from build123d import *

# Parameters (mm, degrees)
SKETCH1_R             = 11
EXTRUDE1_DEPTH        = 2.5
F_6_32_TAPPED_HOLE3_D = 2.7051
CHAMFER1_SIZE         = 0.254
SKETCH2_R             = 4
EXTRUDE2_DEPTH        = 6


with BuildPart() as part:
    # Sketch1 → Extrude1 (new body, symmetric)
    with BuildSketch(Plane.XY):
        Circle(SKETCH1_R)
    extrude(amount=EXTRUDE1_DEPTH, both=True)

    # #6-32 Tapped Hole3 (through all)
    with Locations(Plane(origin=(0, 7.599342077, 2.5), x_dir=(1, 0, 0), z_dir=(0, 0, 1))):
        with Locations((0, 0), (-7.599342077, -7.599342077), (7.599342077, -7.599342077), (0, -15.198684154)):
            Hole(F_6_32_TAPPED_HOLE3_D / 2)

    # Chamfer1
    chamfer1_edges = [part.edges().sort_by_distance(p)[0] for p in [
        (8.951892077, 0, 2.5),
        (8.951892077, 0, -2.5),
        (-6.246792077, 0, 2.5),
        (-6.246792077, 0, -2.5),
        (1.35255, 7.599342077, 2.5),
        (1.35255, 7.599342077, -2.5),
        (1.35255, -7.599342077, 2.5),
        (1.35255, -7.599342077, -2.5),
    ]]
    chamfer(chamfer1_edges, length=CHAMFER1_SIZE)

    # Sketch2 → Extrude2 (cut, through all)
    with BuildSketch(Plane.XY.offset(2.5)):
        Circle(SKETCH2_R)
    extrude(amount=-EXTRUDE2_DEPTH, mode=Mode.SUBTRACT)


solid = part.part
Read the model definition and answer for the solid it produces. Units are mm, in the model's axes. Round coordinates to 2 decimals unless told otherwise and drop trailing zeros. Write each loop counter-clockwise with the first axis right and the second up, starting at its lowest first coordinate (ties: lowest second). Pieces come first, ordered by that corner, then holes.
Q1. Find section C-C on y = -2.5. Determine the outline of the cut face in (x, z).
Values:
outline: (-10.71, -2.5) - (-3.12, -2.5) - (-3.12, 2.5) - (-10.71, 2.5) - close; (3.12, -2.5) - (10.71, -2.5) - (10.71, 2.5) - (3.12, 2.5) - close
Q2. The mould has two halves that part along Y. Classify faces 1 (the face through (-2.38, -10.74, 0.04)), 2 (the face through (0.29, 6.28, -0.03)), 3 (the face through (0, -5, 2.5)): released by +Y, released by -Y, zero draft, split by the parting line, or undercut.
Values:
face 1: split by the parting line
face 2: undercut
face 3: zero draft
Q3. Straight lines are drawn through the part: line 1 (Y direction, x = 0, z = 1.45); line 2 (Y direction, x = -7.5, z = -0.2); line 3 (Y direction, x = -1, z = 0.7). For each, find the intervals that lie inside material, in ascending order.
Values:
line 1: y = -11 to -8.95, -6.25 to -4, 4 to 6.25, 8.95 to 11
line 2: y = -8.05 to -1.35, 1.35 to 8.05
line 3: y = -10.95 to -8.51, -6.69 to -3.87, 3.87 to 6.69, 8.51 to 10.95
Q4. Flat-ended cylindrical pins translate along their axes: P1, Ø1, axis at y = -7.5, z = 0.5, coming from the +X side; P2, Ø1, axis at x = -8.5, y = 0, coming from the -Z side; P3, Ø3, axis at x = -7.6, y = 0, coming from the -Z side. Find the tip coordinate at first contact, or state that the pin passes through.
Values:
P1: stops at x = 8.49
P2: stops at z = -2.29
P3: stops at z = -2.39
Q5. Find section A-A on y = 0. Determine the outline of the cut face in (x, z).
Values:
outline: (-11, -2.5) - (-9.21, -2.5) - (-8.95, -2.25) - (-8.95, 2.25) - (-9.21, 2.5) - (-11, 2.5) - close; (-6.25, -2.25) - (-5.99, -2.5) - (-4, -2.5) - (-4, 2.5) - (-5.99, 2.5) - (-6.25, 2.25) - close; (4, -2.5) - (5.99, -2.5) - (6.25, -2.25) - (6.25, 2.25) - (5.99, 2.5) - (4, 2.5) - close; (8.95, -2.25) - (9.21, -2.5) - (11, -2.5) - (11, 2.5) - (9.21, 2.5) - (8.95, 2.25) - close
Q6. Find section D-D on z = 0.45. Determine the outline of the cut face in (x, y).
Values:
outline: circle Ø22 at (0, 0); hole circle Ø2.71 at (-7.6, 0); hole circle Ø8 at (0, 0); hole circle Ø2.71 at (0, -7.6); hole circle Ø2.71 at (0, 7.6); hole circle Ø2.71 at (7.6, 0)
